```python
from build123d import *

# Parameters (mm, degrees)
SKETCH_1_W          = 38
SKETCH_1_H          = 38
SKETCH_1_R          = 1
EXTRUDE_1_DEPTH     = 1.5
SKETCH_2_R          = 0.75
EXTRUDE_2_DEPTH     = 3.7
SKETCH1_R           = 8
BOSS_EXTRUDE1_DEPTH = 7.7
RIB1_REACH          = 31.806
SKETCH4_WALL_W      = 67.73123823
SKETCH4_WALL_H      = 1
CIRPATTERN1_COUNT   = 10


with BuildPart() as part:
    # 草图1 → 凸台-拉伸1 (new body)
    with BuildSketch(Plane(origin=(0, 0, 0), x_dir=(1, 0, 0), z_dir=(0, 1, 0))):
        Rectangle(SKETCH_1_W, SKETCH_1_H)
        with Locations(Location((-17, 17, 0), (0, 0, 270))):
            Circle(SKETCH_1_R, mode=Mode.SUBTRACT)
        with Locations(Location((17, 17, 0), (0, 0, 90))):
            Circle(SKETCH_1_R, mode=Mode.SUBTRACT)
        with Locations(Location((17, -17, 0), (0, 0, 270))):
            Circle(SKETCH_1_R, mode=Mode.SUBTRACT)
        with Locations(Location((-17, -17, 0), (0, 0, 90))):
            Circle(SKETCH_1_R, mode=Mode.SUBTRACT)
    extrude(amount=EXTRUDE_1_DEPTH)

    # 草图2 → 凸台-拉伸2 (add)
    with BuildSketch(Plane(origin=(0, 1.5, 0), x_dir=(1, 0, 0), z_dir=(0, 1, 0))):
        with BuildLine():
            Line((-10, -10), (10, -10))
            Line((10, -10), (10, -1.5))
            Line((10, -1.5), (11, -1.5))
            ThreePointArc((11, -1.5), (12.5, 0), (11, 1.5))
            Line((11, 1.5), (10, 1.5))
            Line((10, 1.5), (10, 10))
            Line((10, 10), (-10, 10))
            Line((-10, 10), (-10, 1.5))
            Line((-10, 1.5), (-11, 1.5))
            ThreePointArc((-11, 1.5), (-12.5, 0), (-11, -1.5))
            Line((-11, -1.5), (-10, -1.5))
            Line((-10, -1.5), (-10, -10))
        make_face()
        with Locations(Location((11, 0, 0), (0, 0, 270))):
            Circle(SKETCH_2_R, mode=Mode.SUBTRACT)
        with Locations(Location((-11, 0, 0), (0, 0, 90))):
            Circle(SKETCH_2_R, mode=Mode.SUBTRACT)
    extrude(amount=EXTRUDE_2_DEPTH)

    # Sketch1 → Boss-Extrude1 (add)
    with BuildSketch(Plane(origin=(0, 5.2, 0), x_dir=(1, 0, 0), z_dir=(0, 1, 0))):
        with Locations(Location((0, 0, 0), (0, 0, 90))):
            Circle(SKETCH1_R)
    extrude(amount=BOSS_EXTRUDE1_DEPTH)

    # Sketch4 wall → Rib1 (add, up to next)
    with BuildSketch(Plane(origin=(0, 8.2, -8.6), x_dir=(0, -0.980580675691, -0.196116135138), z_dir=(0, 0.196116135138, -0.980580675691)), mode=Mode.PRIVATE) as rib1_sk1:
        Rectangle(SKETCH4_WALL_W, SKETCH4_WALL_H)
    rib1_tool1 = extrude(rib1_sk1.sketch, amount=-RIB1_REACH, mode=Mode.PRIVATE) - part.part
    rib1 = rib1_tool1.solids().sort_by_distance((0, 8.2, -8.6))[0]
    add(rib1)

    # CirPattern1: Rib1 ×10 about axis
    cirpattern1_axis = Axis((0, 0, 0), (0, 1, 0))
    for i in range(1, CIRPATTERN1_COUNT):
        add(rib1.rotate(cirpattern1_axis, i * 360 / CIRPATTERN1_COUNT))

    # Sketch5 → Revolve1 (revolve)
    with BuildSketch(Plane(origin=(0, 0, 0), x_dir=(0, 0, -1), z_dir=(1, 0, 0))):
        Polygon((0, 23.9), (7, 23.9), (7, 19.9), (6.5, 19.9), (6.5, 12.9), (0, 12.9), align=None)
    revolve(axis=Axis((0, 12.9, 0), (0, 1, 0)))


solid = part.part
```
CAD build for the part. Positions are in the model's coordinates, mm. A direction names the side the tool comes from. Coordinates: 2 decimals unless noted, no trailing zeros. Loops run counter-clockwise (first coordinate to the right, second up) from the corner with the lowest first, then second, coordinate; pieces in that order, holes last. Notation, with made-up numbers: (59.25, 22.5) - (113.25, 22.5) arc R23 cw to (113.25, 46.5) - close; hole circle Ø8 at (70, -20). An arc over 180 degrees is marked (long way). Use CSV: the item, a comma, the result in double quotes. Start each with the question number.
Q1. Cut at B-B, the plane y = 4.5. List the corners of the cut face in (x, z).
Q2. Two-plate mould, pull along X, no slides. Class faces 5 (the flat face through (-5.1, 8.3, -6.9)), 6 (the flat face through (8.02, 7.52, -2.08)), 7 (the flat face through (7.71, 7.52, -3.03)): +X half, -X half, draft (parallel to the pull), parting line (faces both ways), or undercut.
Q3. Probe probe 1 along X at (y, z) = (0.5, -17); probe 2 along Z at (x, y) = (5.5, 6.25); probe 3 along Y at (x, z) = (-9, -11.5). List the from-to ranges inside material, lowest first. Write a range as from..to.
Q4. 3-axis set-ups, long thin cutter, end or side, ignore diameter. For faces 1 (the flat face through (10, 3, 6)), 2 (the flat face through (11, 1.5, 0)), 3 (the cylindrical face through (3.955, 16.351, 5.158)), 4 (the flat face through (-10, 3, -6)): which of +Z, -Z, +X, -X, +Y, -Y reach the whole face in a straight line?
Q5. Drop flat-ended pins along their axis: P1, Ø1, axis at x = 10.5, y = 8, coming from the -Z side; P2, Ø8, axis at y = 7.5, z = 7.5, coming from the +X side; P3, Ø0.8, axis at x = 11, z = 0, coming from the +Y side; P4, Ø6, axis at x = 3, y = 12.5, coming from the -Z side. Give the stop position or say it passes through.
Q6. Cut at D-D, the plane x = 0. List the corners of the cut face in (y, z), then the cut area to 3 significant figures.
Q7. Cut at C-C, the plane z = -17. List the corners of the cut face in (x, y).
Q8. Cut at A-A, the plane x = -17. List the corners of the cut face in (y, z).
Here are the results:
1,outline,"(-11, -1.5) - (-10, -1.5) - (-10, -10) - (10, -10) - (10, -1.5) - (11, -1.5) arc R1.5 ccw to (11, 1.5) - (10, 1.5) - (10, 10) - (-10, 10) - (-10, 1.5) - (-11, 1.5) arc R1.5 ccw to start; hole circle Ø1.5 at (-11, 0); hole circle Ø1.5 at (11, 0)"
2,face 5,"-X half"
2,face 6,"+X half"
2,face 7,"undercut"
3,probe 1,"-19..-18, -16..16, 18..19"
3,probe 2,"-7.12..-6.72, -5.81..5.81, 6.72..7.12"
3,probe 3,"0..1.5"
4,face 1,"+Z, +X, +Y"
4,face 2,"+Y"
4,face 3,"none"
4,face 4,"-Z, -X, +Y"
5,P1,"through"
5,P2,"x = 10"
5,P3,"y = 1.5"
5,P4,"z = -8.07"
6,outline,"(0, -19) - (1.5, -19) - (1.5, -10) - (5.2, -10) - (5.2, -9.2) - (11.2, -8) - (12.9, -8) - (12.9, -6.5) - (19.9, -6.5) - (19.9, -7) - (23.9, -7) - (23.9, 7) - (19.9, 7) - (19.9, 6.5) - (12.9, 6.5) - (12.9, 8) - (11.2, 8) - (5.2, 9.2) - (5.2, 10) - (1.5, 10) - (1.5, 19) - (0, 19) - close"
6,area,"408 mm2"
7,outline,"(-19, 0) - (-18, 0) - (-18, 1.5) - (-19, 1.5) - close; (-16, 0) - (16, 0) - (16, 1.5) - (-16, 1.5) - close; (18, 0) - (19, 0) - (19, 1.5) - (18, 1.5) - close"
8,outline,"(0, -19) - (1.5, -19) - (1.5, -18) - (0, -18) - close; (0, -16) - (1.5, -16) - (1.5, 16) - (0, 16) - close; (0, 18) - (1.5, 18) - (1.5, 19) - (0, 19) - close"
